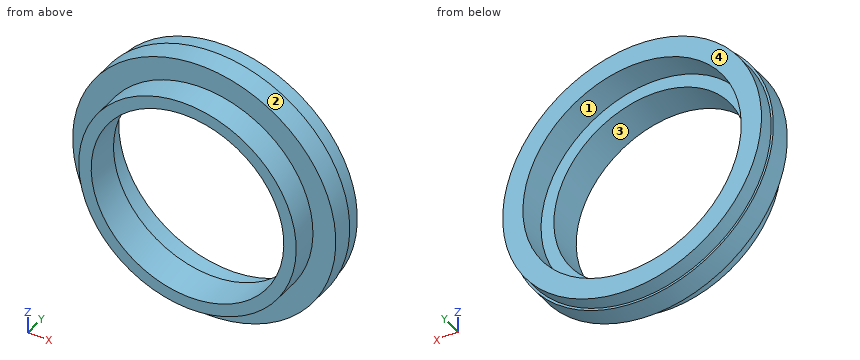
```python
from build123d import *

# Parameters (mm, degrees)
SKETCH1_R           = 12.7
SKETCH1_R_2         = 11.25
BOSS_EXTRUDE1_DEPTH = 3.048
SKETCH2_R           = 15.367
BOSS_EXTRUDE2_DEPTH = 2.54
SKETCH3_R           = 15.113
BOSS_EXTRUDE3_DEPTH = 1.778
SKETCH4_R           = 11.25
CUT_EXTRUDE1_DEPTH  = 4.318
SKETCH5_R           = 12.75
CUT_EXTRUDE2_DEPTH  = 3.302


with BuildPart() as part:
    # Sketch1 → Boss-Extrude1 (new body)
    with BuildSketch(Plane(origin=(0, 0, 0), x_dir=(1, 0, 0), z_dir=(0, 1, 0))):
        with Locations(Location((0, 0, 0), (0, 0, 90))):
            Circle(SKETCH1_R)
        with Locations(Location((0, 0, 0), (0, 0, 90))):
            Circle(SKETCH1_R_2, mode=Mode.SUBTRACT)
    extrude(amount=BOSS_EXTRUDE1_DEPTH)

    # Sketch2 → Boss-Extrude2 (add)
    with BuildSketch(Plane(origin=(0, 3.048, 0), x_dir=(1, 0, 0), z_dir=(0, 1, 0))):
        with Locations(Location((0, 0, 0), (0, 0, 270))):
            Circle(SKETCH2_R)
    extrude(amount=BOSS_EXTRUDE2_DEPTH)

    # Sketch3 → Boss-Extrude3 (add)
    with BuildSketch(Plane(origin=(0, 5.588, 0), x_dir=(1, 0, 0), z_dir=(0, 1, 0))):
        with Locations(Location((0, 0, 0), (0, 0, 270))):
            Circle(SKETCH3_R)
    extrude(amount=BOSS_EXTRUDE3_DEPTH)

    # Sketch4 → Cut-Extrude1 (cut)
    with BuildSketch(Plane.XZ.offset(-3.048)):
        with Locations(Location((0, 0, 0), (0, 0, 270))):
            Circle(SKETCH4_R)
    extrude(amount=-CUT_EXTRUDE1_DEPTH, mode=Mode.SUBTRACT)

    # Sketch5 → Cut-Extrude2 (cut)
    with BuildSketch(Plane(origin=(0, 7.366, 0), x_dir=(1, 0, 0), z_dir=(0, 1, 0))):
        with Locations(Location((0, 0, 0), (0, 0, 270))):
            Circle(SKETCH5_R)
    extrude(amount=-CUT_EXTRUDE2_DEPTH, mode=Mode.SUBTRACT)


solid = part.part
```
Geometry check sheet. Reference: the model listing, model coordinates, mm. Face numbers are marked on the shaded views. Give positions to 0.01 mm unless a question says otherwise; leave off trailing zeros. Order: outer loops, then holes, each group sorted by start corner. A loop starts at its lowest first (then second) coordinate and runs counter-clockwise, first axis right, second up.
1. Section check A-A, the plane z = 0. Enter the section's corners in (x, y).
2. Release check for a two-part mould opening along Z. For the marked faces 1, 2, 3 and 4 record: pulls with the +Z half, pulls with the -Z half, needs draft (parallel to the pull), parting line crosses it, or undercut.
3. Section check D-D, the plane y = 7. Enter the section's corners in (x, z).
4. Section check C-C, the plane y = 4.5. Enter the section's corners in (x, z), and give its area (3 significant figures).
5. Section check B-B, the plane x = 0. Enter the section's corners in (y, z).
6. Thickness scan on L1, parallel to X at y = 1.65, z = 0; L2, parallel to X at y = 6.45, z = 0; L3, parallel to Y at x = -14, z = -4.5. Record the ranges inside material, lowest first.
7. Gauge pin test, flat ends, axial feed: pin 1 Ø1 at (y, z) = (4.5, 5.5) entering from +X; pin 2 Ø1.5 at (y, z) = (1.5, -3.5) entering from -X; pin 3 Ø1 at (y, z) = (5.5, -6.5) entering from +X. Record the tip position at first contact, or that the pin passes through.
Values follow:
1. outline: (-15.37, 3.05) - (-12.7, 3.05) - (-12.7, 0) - (-11.25, 0) - (-11.25, 4.06) - (-12.75, 4.06) - (-12.75, 7.37) - (-15.11, 7.37) - (-15.11, 5.59) - (-15.37, 5.59) - close; (11.25, 0) - (12.7, 0) - (12.7, 3.05) - (15.37, 3.05) - (15.37, 5.59) - (15.11, 5.59) - (15.11, 7.37) - (12.75, 7.37) - (12.75, 4.06) - (11.25, 4.06) - close
2. face 1: undercut
2. face 2: parting line crosses it
2. face 3: undercut
2. face 4: needs draft
3. outline: circle Ø30.23 at (0, 0); hole circle Ø25.5 at (0, 0)
4. outline: circle Ø30.73 at (0, 0); hole circle Ø25.5 at (0, 0)
4. area: 231 mm2
5. outline: (0, -12.7) - (3.05, -12.7) - (3.05, -15.37) - (5.59, -15.37) - (5.59, -15.11) - (7.37, -15.11) - (7.37, -12.75) - (4.06, -12.75) - (4.06, -11.25) - (0, -11.25) - close; (0, 11.25) - (4.06, 11.25) - (4.06, 12.75) - (7.37, 12.75) - (7.37, 15.11) - (5.59, 15.11) - (5.59, 15.37) - (3.05, 15.37) - (3.05, 12.7) - (0, 12.7) - close
6. L1: x = -12.7 to -11.25, 11.25 to 12.7
6. L2: x = -15.11 to -12.75, 12.75 to 15.11
6. L3: y = 3.05 to 7.37
7. pin 1: stops at x = 14.53
7. pin 2: stops at x = -12.4
7. pin 3: stops at x = 14.15
